Work out the finished part from the listing and answer in its coordinate system (mm). A direction names the side the tool comes from. Give positions to 0.01 mm unless a question says otherwise; leave off trailing zeros. Write each loop counter-clockwise with the first axis right and the second up, starting at its lowest first coordinate (ties: lowest second). Pieces come first, ordered by that corner, then holes. Notation, with made-up numbers: (-6, 88.5) - (27, 88.5) arc R9 cw to (27, 92.5) - close; hole circle Ø8 at (77, -27). An arc over 180 degrees is marked (long way). Write item = value, one per line.
from build123d import *

# Parameters (mm, degrees)
SKETCH1_W           = 22.5
SKETCH1_H           = 17.2
BOSS_EXTRUDE1_DEPTH = 1.5
SKETCH2_W           = 1.6
SKETCH2_H           = 3.2
BOSS_EXTRUDE2_DEPTH = 1.5
SKETCH2_3_W         = 5
SKETCH2_3_H         = 3.9
BOSS_EXTRUDE3_DEPTH = 1.3
SKETCH3_W           = 5.6
SKETCH3_H           = 7.5
BOSS_EXTRUDE4_DEPTH = 2.2
SKETCH4_R           = 0.8
CUT_EXTRUDE1_DEPTH  = 16.657346518


with BuildPart() as part:
    # Sketch1 → Boss-Extrude1 (new body)
    with BuildSketch(Plane(origin=(0, 0, 0), x_dir=(1, 0, 0), z_dir=(0, 1, 0))):
        Rectangle(SKETCH1_W, SKETCH1_H)
    extrude(amount=BOSS_EXTRUDE1_DEPTH)

    # Sketch2 → Boss-Extrude2 (add)
    with BuildSketch(Plane(origin=(0, 1.5, 0), x_dir=(1, 0, 0), z_dir=(0, 1, 0))):
        with Locations((0.614877172, -3.370237047)):
            Rectangle(SKETCH2_W, SKETCH2_H)
        with Locations((8.482597382, -1.31074558)):
            Rectangle(SKETCH2_W, SKETCH2_H)
    extrude(amount=BOSS_EXTRUDE2_DEPTH)

    # Sketch2_3 → Boss-Extrude3 (add)
    with BuildSketch(Plane(origin=(0, 1.5, 0), x_dir=(1, 0, 0), z_dir=(0, 1, 0))):
        with Locations((4.675193235, -3.396272098)):
            Rectangle(SKETCH2_3_W, SKETCH2_3_H)
    extrude(amount=BOSS_EXTRUDE3_DEPTH)

    # Sketch3 → Boss-Extrude4 (add)
    with BuildSketch(Plane(origin=(0, 1.5, 0), x_dir=(1, 0, 0), z_dir=(0, 1, 0))):
        with Locations((-9.75, 0)):
            Rectangle(SKETCH3_W, SKETCH3_H)
    extrude(amount=BOSS_EXTRUDE4_DEPTH)

    # Sketch4 → Cut-Extrude1 (cut, through all)
    with BuildSketch(Plane(origin=(0, 0, 0), x_dir=(1, 0, 0), z_dir=(0, 1, 0))):
        with Locations(Location((-9.15, 6.8, 0), (0, 0, 90))):
            Circle(SKETCH4_R)
        with Locations(Location((-9.15, -6.8, 0), (0, 0, 90))):
            Circle(SKETCH4_R)
        with Locations(Location((9.15, -6.8, 0), (0, 0, 90))):
            Circle(SKETCH4_R)
        with Locations(Location((9.15, 6.8, 0), (0, 0, 90))):
            Circle(SKETCH4_R)
    extrude(amount=CUT_EXTRUDE1_DEPTH, mode=Mode.SUBTRACT)


solid = part.part
1. Given pin 1 (0.7 mm diameter, centred on y = 3, z = -1, fed in from +X); pin 2 (0.7 mm diameter, centred on x = -12, z = -0.5, fed in from -Y); pin 3 (4.5 mm diameter, centred on x = 5.5, z = 3, fed in from +Y); pin 4 (1.4 mm diameter, centred on x = 9.15, z = -6.8, fed in from -Y), each flat-ended and moving along its own axis, determine where each tip first touches the part or whether it passes through.
Solution:
pin_1 = -6.95
pin_2 = 1.5
pin_3 = 3
pin_4 = through
2. For a pull along Z with two mould halves and no side action, classify faces 1 (the flat face through (-12.55, 3, 0)), 2 (the flat face through (8, 2, 2.911)), 3 (the cylindrical face through (9.456, 0.74, 6.061)) as pulls with the +Z half, pulls with the -Z half, needs draft (parallel to the pull), parting line crosses it, or undercut.
Solution:
face_1 = needs draft
face_2 = pulls with the +Z half
face_3 = undercut
3. Find section C-C, the plane z = 6.8. Give the vertices of the cut face in (x, y).
Solution:
outline = (-11.25, 0) - (-9.95, 0) - (-9.95, 1.5) - (-11.25, 1.5) - close; (-8.35, 0) - (8.35, 0) - (8.35, 1.5) - (-8.35, 1.5) - close; (9.95, 0) - (11.25, 0) - (11.25, 1.5) - (9.95, 1.5) - close
4. Find section D-D, the plane z = 4. Give the vertices of the cut face in (x, y).
Solution:
outline = (-11.25, 0) - (11.25, 0) - (11.25, 1.5) - (7.18, 1.5) - (7.18, 2.8) - (2.18, 2.8) - (2.18, 1.5) - (1.41, 1.5) - (1.41, 3) - (-0.19, 3) - (-0.19, 1.5) - (-11.25, 1.5) - close
5. Straight lines are drawn through the part: line 1 (X direction, y = 0.45, z = 6.8); line 2 (Z direction, x = 9.15, y = 0.55); line 3 (Y direction, x = 5.5, z = 1.25). For each, find the intervals that lie inside material, in ascending order.
Solution:
line_1 = -11.25 to -9.95, -8.35 to 8.35, 9.95 to 11.25
line_2 = -8.6 to -7.6, -6 to 6, 7.6 to 8.6
line_3 = 0 to 1.5
6. A tool of negligible diameter and unlimited length cuts with its end or side. For faces 4 (the flat face through (9.283, 2, 1)), 5 (the flat face through (-10, 3, 3.75)), 6 (the flat face through (5, 2, 1.446)), from which of +Z, -Z, +X, -X, +Y, -Y can it reach the whole face along a straight path? Write none if from no direction.
Solution:
face_4 = +Z, -Z, +X, +Y
face_5 = +Z, -X, +Y
face_6 = -Z, +Y
7. Find section A-A, the plane y = 2.45. Give the vertices of the cut face in (x, z).
Solution:
outline = (-12.55, -3.75) - (-6.95, -3.75) - (-6.95, 3.75) - (-12.55, 3.75) - close; (-0.19, 1.77) - (1.41, 1.77) - (1.41, 4.97) - (-0.19, 4.97) - close; (2.18, 1.45) - (7.18, 1.45) - (7.18, 5.35) - (2.18, 5.35) - close; (7.68, -0.29) - (9.28, -0.29) - (9.28, 2.91) - (7.68, 2.91) - close
8. Find section B-B, the plane x = -9.15. Give the vertices of the cut face in (y, z), then the cut area to 3 significant figures.
Solution:
outline = (0, -8.6) - (1.5, -8.6) - (1.5, -7.6) - (0, -7.6) - close; (0, -6) - (1.5, -6) - (1.5, -3.75) - (3.7, -3.75) - (3.7, 3.75) - (1.5, 3.75) - (1.5, 6) - (0, 6) - close; (0, 7.6) - (1.5, 7.6) - (1.5, 8.6) - (0, 8.6) - close
area = 37.5 mm^2
